Work out the finished part from the listing and answer in its coordinate system (mm). Face numbers are marked on the shaded views. A direction names the side the tool comes from. Coordinates: 2 decimals unless noted, no trailing zeros. Order: outer loops, then holes, each group sorted by start corner. A loop starts at its lowest first (then second) coordinate and runs counter-clockwise, first axis right, second up. Notation, with made-up numbers: (73, -36.5) -> (95, -36.5) arc R14 ccw to (95, -25.5) -> close; hole circle Ø11 at (51, 26). An arc over 180 degrees is marked (long way). Write item = value, one per line. Start each with the question number.
Q1. The part is cut by section C-C, the plane z = 84.5. Determine the outline of the cut face in (x, y), plus the area to 3 significant figures.
Q2. The part is cut by section D-D, the plane z = 178. Determine the outline of the cut face in (x, y).
Q3. Straight lines are drawn through the part: L1, parallel to Y at x = 0, z = 191; L2, parallel to Z at x = 20.5, y = -27.5; L3, parallel to Z at x = -4, y = 16. For each, find the intervals that lie inside material, in ascending order. Write a range as from..to.
Q4. Which of the six approach directions +Z, -Z, +X, -X, +Y, -Y give full straight-line access (tool end or side, diameter ignored) to the marked faces 1 and 2?
Q5. The part is cut by section A-A, the plane x = 32. Determine the outline of the cut face in (y, z).
Q6. The part is cut by section B-B, the plane y = 32. Determine the outline of the cut face in (x, z).
Q7. Flat-ended cylindrical pins translate along their axes: pin 1 (8 mm diameter, centred on x = -2, y = 17.5, fed in from +Z); pin 2 (2 mm diameter, centred on x = 10.5, y = 9.5, fed in from +Z); pin 3 (10 mm diameter, centred on x = -9.5, z = 127, fed in from +Y); pin 4 (3 mm diameter, centred on x = 9.5, z = 152.5, fed in from +Y). Find the tip coordinate at first contact, or state that the pin passes through.
```python
from build123d import *

# Parameters (mm, degrees)
SKETCH_1_R          = 20
EXTRUDE_1_DEPTH     = 180
SKETCH_3_R          = 37
EXTRUDE_3_DEPTH     = 16
SKETCH_4_R          = 20.5
CUT_EXTRUDE_1_DEPTH = 6
SKETCH_5_R          = 9.75
EXTRUDE_4_DEPTH     = 6
CUT_EXTRUDE_3_REACH = 198
SKETCH_10_R         = 2.45
SKETCH_18_R         = 4.4
CUT_EXTRUDE_4_DEPTH = 5


with BuildPart() as part:
    # 스케치1 → 보스-돌출1 (new body)
    with BuildSketch(Plane.XY):
        Circle(SKETCH_1_R)
    extrude(amount=EXTRUDE_1_DEPTH)

    # 스케치3 → 보스-돌출3 (add)
    with BuildSketch(Plane.XY.offset(180)):
        Circle(SKETCH_3_R)
    extrude(amount=EXTRUDE_3_DEPTH)

    # 스케치4 → 컷-돌출1 (cut)
    with BuildSketch(Plane.XY.offset(196)):
        Circle(SKETCH_4_R)
    extrude(amount=-CUT_EXTRUDE_1_DEPTH, mode=Mode.SUBTRACT)

    # 스케치5 → 보스-돌출4 (add)
    with BuildSketch(Plane.XY.offset(190)):
        Circle(SKETCH_5_R)
    extrude(amount=EXTRUDE_4_DEPTH)

    # 스케치10 → 컷-돌출3 (cut, up to next)
    with BuildSketch(Plane.XY.offset(196), mode=Mode.PRIVATE) as cut_extrude_3_sk1:
        with Locations((0, 32)):
            Circle(SKETCH_10_R)
    cut_extrude_3_tool1 = extrude(cut_extrude_3_sk1.sketch, amount=-CUT_EXTRUDE_3_REACH, mode=Mode.PRIVATE) & part.part
    add(cut_extrude_3_tool1.solids().sort_by_distance((0, 32, 196))[0], mode=Mode.SUBTRACT)
    # 스케치10 → 컷-돌출3 (cut, up to next)
    with BuildSketch(Plane.XY.offset(196), mode=Mode.PRIVATE) as cut_extrude_3_sk2:
        with Locations((32, 0.150294809)):
            Circle(SKETCH_10_R)
    cut_extrude_3_tool2 = extrude(cut_extrude_3_sk2.sketch, amount=-CUT_EXTRUDE_3_REACH, mode=Mode.PRIVATE) & part.part
    add(cut_extrude_3_tool2.solids().sort_by_distance((32, 0.150295, 196))[0], mode=Mode.SUBTRACT)
    # 스케치10 → 컷-돌출3 (cut, up to next)
    with BuildSketch(Plane.XY.offset(196), mode=Mode.PRIVATE) as cut_extrude_3_sk3:
        with Locations((-32, 0.258434211)):
            Circle(SKETCH_10_R)
    cut_extrude_3_tool3 = extrude(cut_extrude_3_sk3.sketch, amount=-CUT_EXTRUDE_3_REACH, mode=Mode.PRIVATE) & part.part
    add(cut_extrude_3_tool3.solids().sort_by_distance((-32, 0.258434, 196))[0], mode=Mode.SUBTRACT)
    # 스케치10 → 컷-돌출3 (cut, up to next)
    with BuildSketch(Plane.XY.offset(196), mode=Mode.PRIVATE) as cut_extrude_3_sk4:
        with Locations((-0.108139402, -32)):
            Circle(SKETCH_10_R)
    cut_extrude_3_tool4 = extrude(cut_extrude_3_sk4.sketch, amount=-CUT_EXTRUDE_3_REACH, mode=Mode.PRIVATE) & part.part
    add(cut_extrude_3_tool4.solids().sort_by_distance((-0.108139, -32, 196))[0], mode=Mode.SUBTRACT)

    # 스케치18 → 컷-돌출4 (cut)
    with BuildSketch(Plane(origin=(0, 0, 180), x_dir=(-1, 0, 0), z_dir=(0, 0, -1))):
        with Locations((0, 32)):
            Circle(SKETCH_18_R)
        with Locations((32, 0.258434211)):
            Circle(SKETCH_18_R)
        with Locations((0.108139402, -32)):
            Circle(SKETCH_18_R)
        with Locations((-32, 0.150294809)):
            Circle(SKETCH_18_R)
    extrude(amount=-CUT_EXTRUDE_4_DEPTH, mode=Mode.SUBTRACT)

    # 스케치20 → 회전1 (revolve)
    with BuildSketch(Plane(origin=(0, 0, 0), x_dir=(1, 0, 0), z_dir=(0, 1, 0))):
        Polygon((-20, -180), (-27.6, -180), (-20, -165), align=None)
    revolve(axis=Axis((0, 0, 180), (0, 0, -1)))


solid = part.part
```
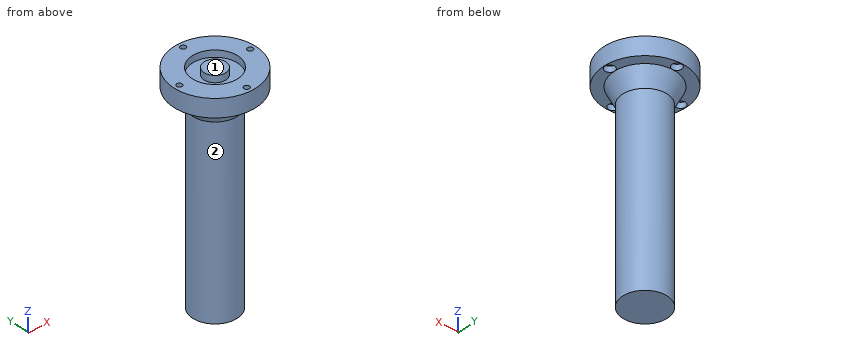
Model answer:
q1.outline = circle Ø40 at (0, 0)
q1.area = 1,260 mm2
q2.outline = circle Ø53.17 at (0, 0)
q3.L1 = -37..-34.45, -29.55..-20.5, -9.75..9.75, 20.5..29.55, 34.45..37
q3.L2 = 180..196
q3.L3 = 0..190
q4.face_1 = +Z, +X, -X, +Y, -Y
q4.face_2 = -Z
q5.outline = (-18.57, 180) -> (-4.25, 180) -> (-4.25, 185) -> (-2.3, 185) -> (-2.3, 196) -> (-18.57, 196) -> close; (2.6, 185) -> (4.55, 185) -> (4.55, 180) -> (18.57, 180) -> (18.57, 196) -> (2.6, 196) -> close
q6.outline = (-18.57, 180) -> (-4.4, 180) -> (-4.4, 185) -> (-2.45, 185) -> (-2.45, 196) -> (-18.57, 196) -> close; (2.45, 185) -> (4.4, 185) -> (4.4, 180) -> (18.57, 180) -> (18.57, 196) -> (2.45, 196) -> close
q7.pin_1 = 196
q7.pin_2 = 190
q7.pin_3 = 19.49
q7.pin_4 = 18.33
